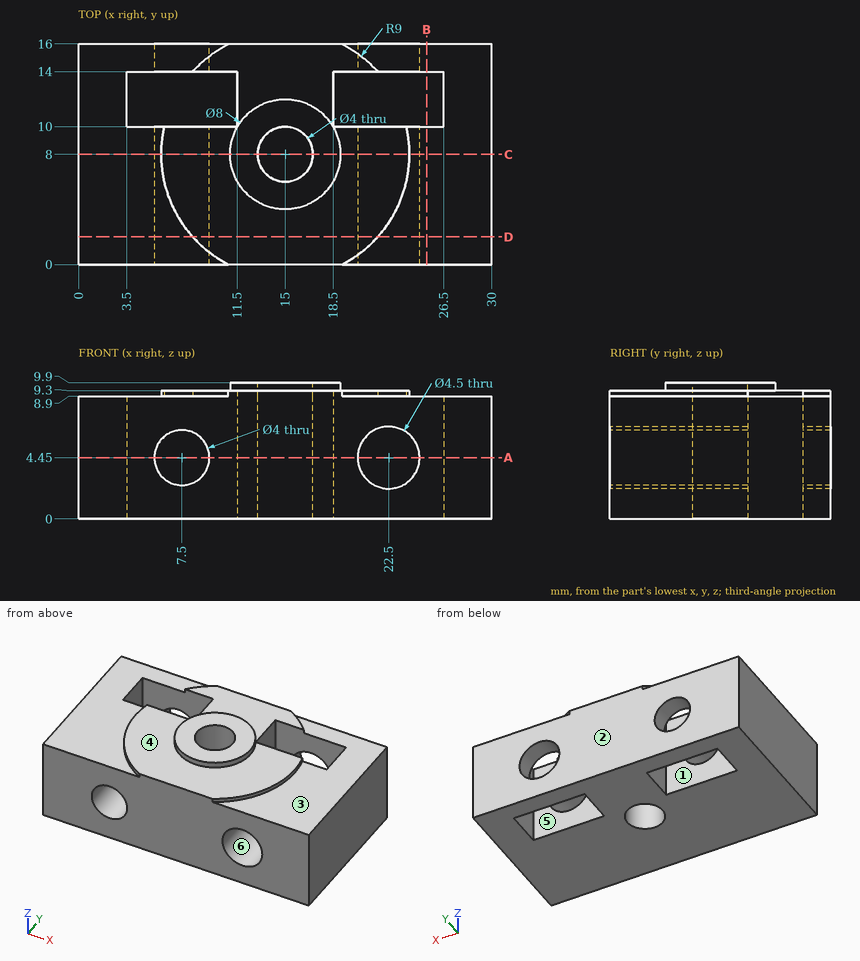
Study the drawing (mm; zero at the part's minimum x, y, z) and answer. A direction names the side the tool comes from. Round coordinates to 2 decimals unless told otherwise and drop trailing zeros. Write each loop counter-clockwise with the first axis right and the second up, starting at its lowest first coordinate (ties: lowest second). Pieces come first, ordered by that corner, then holes.
1) A cutting plane is placed at C-C on y = 8. Determine the outline of the cut face in (x, z).
2) Which of the six approach directions +Z, -Z, +X, -X, +Y, -Y give full straight-line access (tool end or side, diameter ignored) to the marked faces 4, 5 and 6?
3) A cutting plane is placed at D-D on y = 2. Determine the outline of the cut face in (x, z), and give its area (3 significant figures).
4) A flat-ended cylindrical pin translates along its axis: P1, Ø5.5, axis at x = 26.5, y = 8.5, coming from the +Z side. Find the tip coordinate at first contact, or state that the pin passes through.
5) A cutting plane is placed at A-A on z = 4.45. Give the number of separate pieces and of enclosed holes in the cut face, and give its area (3 significant figures).
6) Determine the mould class of the marked faces 1, 2 and 3 for opening direction Y: pulls with the +Y half, pulls with the -Y half, needs draft (parallel to the pull), parting line crosses it, or undercut.
7) Consider probe 1 along Y at (x, z) = (7.25, 1.5); probe 2 along Y at (x, z) = (15, 5.25); probe 3 along Z at (x, y) = (7.5, 14.7). Determine where each line is inside the solid, lowest interval first.
8) A cutting plane is placed at B-B on x = 25.25. Determine the outline of the cut face in (y, z), and give its area (3 significant figures).
Entries:
1. outline: (0, 0) - (13, 0) - (13, 9.9) - (11, 9.9) - (11, 9.3) - (6, 9.3) - (6, 8.9) - (0, 8.9) - close; (17, 0) - (30, 0) - (30, 8.9) - (24, 8.9) - (24, 9.3) - (19, 9.3) - (19, 9.9) - (17, 9.9) - close; hole circle Ø4 at (7.5, 4.45); hole circle Ø4.5 at (22.5, 4.45)
2. face 4: +Z
2. face 5: +Z, -Z
2. face 6: +Y, -Y
3. outline: (0, 0) - (30, 0) - (30, 8.9) - (21.71, 8.9) - (21.71, 9.3) - (8.29, 9.3) - (8.29, 8.9) - (0, 8.9) - close; hole circle Ø4 at (7.5, 4.45); hole circle Ø4.5 at (22.5, 4.45)
3. area: 244 mm2
4. P1: stops at z = 9.3
5. separate pieces: 3
5. enclosed holes: 1
5. area: 301 mm2
6. face 1: undercut
6. face 2: pulls with the +Y half
6. face 3: needs draft
7. probe 1: y = 0 to 10, 14 to 16
7. probe 2: y = 0 to 6, 10 to 16
7. probe 3: z = 0 to 2.45, 6.45 to 8.9
8. outline: (0, 0) - (10, 0) - (10, 8.9) - (0, 8.9) - close; (14, 0) - (16, 0) - (16, 8.9) - (14, 8.9) - close
8. area: 107 mm2
